Could you check a few things on this drawing? It's one solid part, dimensions in mm from its lowest x, y, z. A direction names the side the tool comes from. Round coordinates to 2 decimals unless told otherwise and drop trailing zeros. Loops run counter-clockwise (first coordinate to the right, second up) from the corner with the lowest first, then second, coordinate; pieces in that order, holes last. Notation, with made-up numbers: M 17,5 L 26,5 A28 ccw 26,39 Z; hole C 20,-37.5 d10. An arc over 180 degrees is marked long. Return JSON: item names as keys, results as strings.
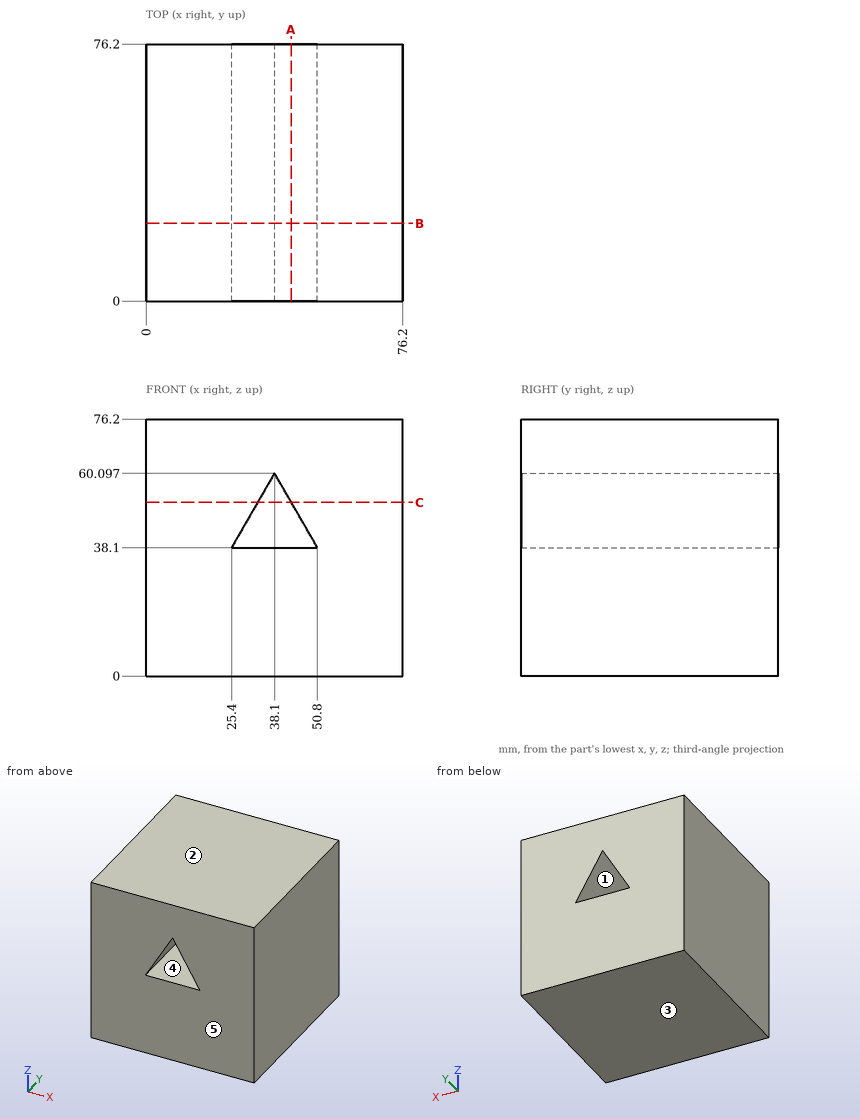
Q1. Thinking about a two-plate mould opening in Z: for the marked faces 3, 4 and 5, which applies, pulls with the +Z half, pulls with the -Z half, needs draft (parallel to the pull), parting line crosses it, or undercut?
Results:
{"face 3": "pulls with the -Z half", "face 4": "undercut", "face 5": "needs draft"}
Q2. If I drill on line 1 along Z through (x, y) = (36.5, 51.5); line 2 along X through (y, z) = (40.5, 44.5) (3 decimals); line 3 along X through (y, z) = (49, 46.5), over which ranges is the centre line in solid material (lowest first)?
Results:
{"line 1": "z = 0 to 38.1, 57.33 to 76.2", "line 2": "x = 0 to 29.095, 47.105 to 76.2", "line 3": "x = 0 to 30.25, 45.95 to 76.2"}
Q3. Suppose I cut it at C-C, the plane z = 51.5. Please give me the cut outline in (x, y).
Results:
{"outline": "M 0,0 L 33.14,0 L 33.14,76.2 L 0,76.2 Z; M 43.06,0 L 76.2,0 L 76.2,76.2 L 43.06,76.2 Z"}
Q4. Suppose I cut it at B-B, the plane y = 23. Please give me the cut outline in (x, z), plus the area to 3 significant figures.
Results:
{"outline": "M 0,0 L 76.2,0 L 76.2,76.2 L 0,76.2 Z; hole M 25.4,38.1 L 50.8,38.1 L 38.1,60.1 Z", "area": "5,530 mm2"}
Q5. Suppose I cut it at A-A, the plane x = 43. Please give me the cut outline in (y, z).
Results:
{"outline": "M 0,0 L 76.2,0 L 76.2,38.1 L 0,38.1 Z; M 0,51.61 L 76.2,51.61 L 76.2,76.2 L 0,76.2 Z"}
Q6. On a 3-axis mill with a long thin cutter (end or side, diameter ignored), from which of +Z, -Z, +X, -X, +Y, -Y can I reach the whole of each face in a straight line? I mean the marked faces 1 and 2. Say none if no direction works.
Results:
{"face 1": "+Y, -Y", "face 2": "+Z, +X, -X, +Y, -Y"}
